Verification items for the finished model (mm, model axes). A direction names the side the tool comes from. Give positions to 0.01 mm unless a question says otherwise; leave off trailing zeros. Order: outer loops, then holes, each group sorted by start corner. A loop starts at its lowest first (then second) coordinate and runs counter-clockwise, first axis right, second up.
from build123d import *

# Parameters (mm, degrees)
SKETCH_1_W        = 30
SKETCH_1_H        = 30
SKETCH_1_W_2      = 26
SKETCH_1_H_2      = 26
EXTRUDE_1_DEPTH   = 200
EXTRUDE_1_2_DEPTH = 200
EXTRUDE_1_3_DEPTH = 200
EXTRUDE_1_4_DEPTH = 200
SKETCH_2_W        = 310
SKETCH_2_H        = 310
EXTRUDE_2_DEPTH   = 3
SKETCH_5_W        = 25
SKETCH_5_H        = 25
SKETCH_5_W_2      = 22
SKETCH_5_H_2      = 22
EXTRUDE_3_DEPTH   = 900
SKETCH_6_W        = 340
SKETCH_6_H        = 340
SKETCH_6_W_2      = 200
SKETCH_6_H_2      = 200
EXTRUDE_4_DEPTH   = 1.5
SKETCH_7_W        = 200
SKETCH_7_H        = 120
EXTRUDE_5_DEPTH   = 1.5
SKETCH_8_W        = 200
SKETCH_8_H        = 1.5
EXTRUDE_6_DEPTH   = 25
SKETCH_9_W        = 200
SKETCH_9_H        = 1.5
EXTRUDE_7_DEPTH   = 25
SKETCH_11_W       = 200
SKETCH_11_H       = 1.5
EXTRUDE_8_DEPTH   = 25
SKETCH_12_W       = 30
SKETCH_12_H       = 30
EXTRUDE_9_DEPTH   = 230
SKETCH_13_W       = 30
SKETCH_13_H       = 30
EXTRUDE_10_DEPTH  = 230
SKETCH_14_W       = 25
SKETCH_14_H       = 25
EXTRUDE_11_DEPTH  = 220
SKETCH_15_W       = 25
SKETCH_15_H       = 25
EXTRUDE_12_DEPTH  = 220


with BuildPart() as part:
    # Sketch 1 → Extrude 1 (new body)
    with BuildSketch(Plane.XY):
        with Locations((-83.068744212, 102.787427317)):
            Rectangle(SKETCH_1_W, SKETCH_1_H)
        with Locations((-83.068744212, 102.787427317)):
            Rectangle(SKETCH_1_W_2, SKETCH_1_H_2, mode=Mode.SUBTRACT)
    extrude(amount=EXTRUDE_1_DEPTH)



with BuildPart() as body_2:
    # Sketch 1 → Extrude 1 2 (new body)
    with BuildSketch(Plane.XY):
        with Locations((176.931255788, 102.787427317)):
            Rectangle(SKETCH_1_W, SKETCH_1_H)
        with Locations((176.931255788, 102.787427317)):
            Rectangle(SKETCH_1_W_2, SKETCH_1_H_2, mode=Mode.SUBTRACT)
    extrude(amount=EXTRUDE_1_2_DEPTH)


with BuildPart() as body_3:
    # Sketch 1 → Extrude 1 3 (new body)
    with BuildSketch(Plane.XY):
        with Locations((-83.068744212, -157.212572683)):
            Rectangle(SKETCH_1_W, SKETCH_1_H)
        with Locations((-83.068744212, -157.212572683)):
            Rectangle(SKETCH_1_W_2, SKETCH_1_H_2, mode=Mode.SUBTRACT)
    extrude(amount=EXTRUDE_1_3_DEPTH)


with BuildPart() as body_4:
    # Sketch 1 → Extrude 1 4 (new body)
    with BuildSketch(Plane.XY):
        with Locations((176.931255788, -157.212572683)):
            Rectangle(SKETCH_1_W, SKETCH_1_H)
        with Locations((176.931255788, -157.212572683)):
            Rectangle(SKETCH_1_W_2, SKETCH_1_H_2, mode=Mode.SUBTRACT)
    extrude(amount=EXTRUDE_1_4_DEPTH)


with BuildPart() as part_1:
    add(part.part)

    add(body_2.part)  # Extrude 2 merges body 2

    add(body_3.part)  # Extrude 2 merges body 3

    add(body_4.part)  # Extrude 2 merges body 4
    # Sketch 2 → Extrude 2 (add)
    with BuildSketch(Plane.XY.offset(200)):
        with Locations((46.931255788, -27.212572683)):
            Rectangle(SKETCH_2_W, SKETCH_2_H)
    extrude(amount=EXTRUDE_2_DEPTH)

    # Sketch 5 → Extrude 3 (add)
    with BuildSketch(Plane.XY.offset(203)):
        with Locations((-65.568744212, 85.287427317)):
            Rectangle(SKETCH_5_W, SKETCH_5_H)
        with Locations((-65.568744212, 85.287427317)):
            Rectangle(SKETCH_5_W_2, SKETCH_5_H_2, mode=Mode.SUBTRACT)
        with Locations((-65.568744212, -139.712572683)):
            Rectangle(SKETCH_5_W, SKETCH_5_H)
        with Locations((-65.568744212, -139.712572683)):
            Rectangle(SKETCH_5_W_2, SKETCH_5_H_2, mode=Mode.SUBTRACT)
        with Locations((159.431255788, -139.712572683)):
            Rectangle(SKETCH_5_W, SKETCH_5_H)
        with Locations((159.431255788, -139.712572683)):
            Rectangle(SKETCH_5_W_2, SKETCH_5_H_2, mode=Mode.SUBTRACT)
        with Locations((159.431255788, 85.287427317)):
            Rectangle(SKETCH_5_W, SKETCH_5_H)
        with Locations((159.431255788, 85.287427317)):
            Rectangle(SKETCH_5_W_2, SKETCH_5_H_2, mode=Mode.SUBTRACT)
    extrude(amount=EXTRUDE_3_DEPTH)

    # Sketch 6 → Extrude 4 (add)
    with BuildSketch(Plane.XY.offset(1103)):
        with Locations((46.931255788, -27.212572683)):
            Rectangle(SKETCH_6_W, SKETCH_6_H)
        with Locations((46.931255788, -27.212572683)):
            Rectangle(SKETCH_6_W_2, SKETCH_6_H_2, mode=Mode.SUBTRACT)
    extrude(amount=EXTRUDE_4_DEPTH)

    # Sketch 7 → Extrude 5 (add)
    with BuildSketch(Plane.XY.offset(573)):
        with Locations((46.931255788, 132.787427317)):
            Rectangle(SKETCH_7_W, SKETCH_7_H)
        with Locations((46.931255788, -187.212572683)):
            Rectangle(SKETCH_7_W, SKETCH_7_H)
    extrude(amount=EXTRUDE_5_DEPTH)

    # Sketch 8 → Extrude 6 (add, symmetric)
    with BuildSketch(Plane(origin=(0, 0, 953), x_dir=(-1, 0, 0), z_dir=(0, 0, -1))):
        with Locations((-46.931255788, 73.537427317)):
            Rectangle(SKETCH_8_W, SKETCH_8_H)
        with Locations((-46.931255788, -127.962572683)):
            Rectangle(SKETCH_8_W, SKETCH_8_H)
    extrude(amount=EXTRUDE_6_DEPTH, both=True)

    # Sketch 9 → Extrude 7 (add, symmetric)
    with BuildSketch(Plane(origin=(0, 0, 741), x_dir=(-1, 0, 0), z_dir=(0, 0, -1))):
        with Locations((-46.931255788, 73.537427317)):
            Rectangle(SKETCH_9_W, SKETCH_9_H)
        with Locations((-46.931255788, -127.962572683)):
            Rectangle(SKETCH_9_W, SKETCH_9_H)
    extrude(amount=EXTRUDE_7_DEPTH, both=True)

    # Sketch 11 → Extrude 8 (add, symmetric)
    with BuildSketch(Plane(origin=(0, 0, 503), x_dir=(-1, 0, 0), z_dir=(0, 0, -1))):
        with Locations((-46.931255788, -127.962572683)):
            Rectangle(SKETCH_11_W, SKETCH_11_H)
        with Locations((-46.931255788, 73.537427317)):
            Rectangle(SKETCH_11_W, SKETCH_11_H)
    extrude(amount=EXTRUDE_8_DEPTH, both=True)

    # Sketch 12 → Extrude 9 (add)
    with BuildSketch(Plane(origin=(-68.068744212, 0, 0), x_dir=(0, 0, -1), z_dir=(1, 0, 0))):
        with Locations((-185, 102.787427317)):
            Rectangle(SKETCH_12_W, SKETCH_12_H)
        with Locations((-185, -157.212572683)):
            Rectangle(SKETCH_12_W, SKETCH_12_H)
    extrude(amount=EXTRUDE_9_DEPTH)

    # Sketch 13 → Extrude 10 (add)
    with BuildSketch(Plane(origin=(0, -142.212572683, 0), x_dir=(1, 0, 0), z_dir=(0, 1, 0))):
        with Locations((-83.068744212, -185)):
            Rectangle(SKETCH_13_W, SKETCH_13_H)
        with Locations((176.931255788, -185)):
            Rectangle(SKETCH_13_W, SKETCH_13_H)
    extrude(amount=EXTRUDE_10_DEPTH)

    # Sketch 14 → Extrude 11 (add)
    with BuildSketch(Plane(origin=(0, -127.212572683, 0), x_dir=(1, 0, 0), z_dir=(0, 1, 0))):
        with Locations((-65.568744212, -1090.5)):
            Rectangle(SKETCH_14_W, SKETCH_14_H)
        with Locations((159.431255788, -1090.5)):
            Rectangle(SKETCH_14_W, SKETCH_14_H)
    extrude(amount=EXTRUDE_11_DEPTH)

    # Sketch 15 → Extrude 12 (add)
    with BuildSketch(Plane(origin=(-53.068744212, 0, 0), x_dir=(0, 0, -1), z_dir=(1, 0, 0))):
        with Locations((-1090.5, 85.287427317)):
            Rectangle(SKETCH_15_W, SKETCH_15_H)
        with Locations((-1090.5, -139.712572683)):
            Rectangle(SKETCH_15_W, SKETCH_15_H)
    extrude(amount=EXTRUDE_12_DEPTH)


solid = part_1.part
(1) Scan lines: line 1 (Z direction, x = 43.5, y = -150); line 2 (Y direction, x = 176, z = 133); line 3 (Z direction, x = 67.5, y = -174). Record each from-to range of solid material in increasing order.
Solved:
line 1: z = 170 to 203, 573 to 574.5, 1078 to 1104.5
line 2: y = -172.21 to -170.21, -144.21 to -142.21, 87.79 to 89.79, 115.79 to 117.79
line 3: z = 200 to 203, 573 to 574.5, 1103 to 1104.5
(2) Release check for a two-part mould opening along X. For faces 1 (the flat face through (189.931, 103, 99)), 2 (the flat face through (-66, -140, 1103)), 3 (the flat face through (68, 117.787, 174)), 4 (the flat face through (171.931, 74, 684)) record: pulls with the +X half, pulls with the -X half, needs draft (parallel to the pull), parting line crosses it, or undercut.
Solved:
face 1: undercut
face 2: undercut
face 3: needs draft
face 4: pulls with the +X half
(3) Section check B-B, the plane y = 21. Enter the section's corners in (x, z), then the cut area to 3 significant figures.
Solved:
outline: (-123.07, 1103) - (-78.07, 1103) - (-78.07, 1078) - (-53.07, 1078) - (-53.07, 1104.5) - (-123.07, 1104.5) - close; (-108.07, 200) - (-98.07, 200) - (-98.07, 170) - (-68.07, 170) - (-68.07, 200) - (161.93, 200) - (161.93, 170) - (191.93, 170) - (191.93, 200) - (201.93, 200) - (201.93, 203) - (-108.07, 203) - close; (146.93, 1078) - (171.93, 1078) - (171.93, 1103) - (216.93, 1103) - (216.93, 1104.5) - (146.93, 1104.5) - close
area: 4,190 mm2
(4) Go/stop test with flat-tipped pins: pin 1 (1.8 mm diameter, centred on x = 168, y = -139.5, fed in from -Z); pin 2 (6.5 mm diameter, centred on x = 156.5, z = 476.5, fed in from -Y); pin 3 (1.5 mm diameter, centred on x = 26, z = 202, fed in from -Y); pin 4 (24 mm diameter, centred on x = 161, y = 83.5, fed in from -Z). Record where each tip stops, or that it passes through.
Solved:
pin 1: stops at z = 170
pin 2: stops at y = -152.21
pin 3: stops at y = -182.21
pin 4: stops at z = 0
(5) Set-up check for faces 5 (the flat face through (177, -29, 170)), 6 (the flat face through (46, 134, 573)), 7 (the flat face through (-54.569, -140, 647)), 8 (the flat face through (-83, 103, 200)), 9 (the flat face through (191.931, -6, 174)): record each of +Z, -Z, +X, -X, +Y, -Y from which the full face is reachable in a straight line by a thin tool's end or side.
Solved:
face 5: -Z, +X, -X
face 6: +Y, -Y
face 7: none
face 8: -Z
face 9: -Z, +X, +Y, -Y
(6) Section check A-A, the plane z = 87.5. Give the number of separate pieces and of enclosed holes in the cut face, then the cut area to 3 significant figures.
Solved:
separate pieces: 4
enclosed holes: 4
area: 896 mm2
